```python
from build123d import *

# Parameters (mm, degrees)
EXTRUDE_1_DEPTH     = 20
SKETCH_2_W          = 12.3
SKETCH_2_H          = 5
CUT_EXTRUDE_1_DEPTH = 12
FILLET_1_R          = 1
FILLET_2_R          = 1.5
CUT_EXTRUDE_5_DEPTH = 21
SKETCH_3_R          = 0.9
CUT_EXTRUDE_2_DEPTH = 8
SKETCH_4_R          = 2
CUT_EXTRUDE_3_DEPTH = 8
CUT_EXTRUDE_4_DEPTH = 8


with BuildPart() as part:
    # 草图1 → 凸台-拉伸1 (new body)
    with BuildSketch(Plane(origin=(0, 0, 0), x_dir=(1, 0, 0), z_dir=(0, 1, 0))):
        with BuildLine():
            Line((-6.15, 0), (-11.5, 0))
            Line((-11.5, 0), (-11.5, 2))
            Line((-11.5, 2), (-8, 2))
            Line((-8, 2), (-8, 6.5))
            Line((-8, 6.5), (8, 6.5))
            Line((8, 6.5), (8, 2))
            Line((8, 2), (11.5, 2))
            Line((11.5, 2), (11.5, 0))
            Line((11.5, 0), (6.15, 0))
            ThreePointArc((6.15, 0), (5.470134317, 2.810717088), (3.580851854, 5))
            Line((3.580851854, 5), (-3.580851854, 5))
            ThreePointArc((-3.580851854, 5), (-5.470134317, 2.810717088), (-6.15, 0))
        make_face()
    extrude(amount=EXTRUDE_1_DEPTH)

    # 草图2 → 切除-拉伸1 (cut)
    with BuildSketch(Plane(origin=(0, 20, 0), x_dir=(1, 0, 0), z_dir=(0, 1, 0))):
        with Locations((0, 2.5)):
            Rectangle(SKETCH_2_W, SKETCH_2_H)
    extrude(amount=-CUT_EXTRUDE_1_DEPTH, mode=Mode.SUBTRACT)

    # 圆角1
    fillet_1_edges = [part.edges().sort_by_distance(p)[0] for p in [
        (-6.15, 14, -5),
        (6.15, 14, -5),
    ]]
    fillet(fillet_1_edges, radius=FILLET_1_R)

    # 圆角2
    fillet_2_edges = [part.edges().sort_by_distance(p)[0] for p in [
        (-8, 10, -2),
        (8, 10, -2),
    ]]
    fillet(fillet_2_edges, radius=FILLET_2_R)

    # 草图6 → 切除-拉伸5 (cut, through all)
    with BuildSketch(Plane(origin=(0, 20, 0), x_dir=(1, 0, 0), z_dir=(0, 1, 0))):
        Polygon((-5.75, 6.5), (-8.528510242, 4.895826364), (-8.528510242, 6.5), align=None)
        Polygon((8.528510242, 6.5), (5.75, 6.5), (8.528510242, 4.895826364), align=None)
    extrude(amount=-CUT_EXTRUDE_5_DEPTH, mode=Mode.SUBTRACT)

    # 草图3 → 切除-拉伸2 (cut)
    with BuildSketch(Plane(origin=(0, 0, -6.5), x_dir=(-1, 0, 0), z_dir=(0, 0, -1))):
        with Locations((-8, 4.5)):
            Circle(SKETCH_3_R)
        with Locations((-8, 15.5)):
            Circle(SKETCH_3_R)
        with Locations((8, 15.5)):
            Circle(SKETCH_3_R)
        with Locations((8, 4.5)):
            Circle(SKETCH_3_R)
    extrude(amount=-CUT_EXTRUDE_2_DEPTH, mode=Mode.SUBTRACT)

    # 草图4 → 切除-拉伸3 (cut)
    with BuildSketch(Plane(origin=(0, 0, -2), x_dir=(-1, 0, 0), z_dir=(0, 0, -1))):
        with Locations((-8, 15.5)):
            Circle(SKETCH_4_R)
        with Locations((-8, 4.5)):
            Circle(SKETCH_4_R)
        with Locations((8, 15.5)):
            Circle(SKETCH_4_R)
        with Locations((8, 4.5)):
            Circle(SKETCH_4_R)
    extrude(amount=CUT_EXTRUDE_3_DEPTH, mode=Mode.SUBTRACT)

    # 草图5 → 切除-拉伸4 (cut)
    with BuildSketch(Plane.XY.offset(-5)):
        with BuildLine():
            Line((-2.5, 17.5), (2.5, 17.5))
            ThreePointArc((2.5, 17.5), (3.207106781, 17.207106781), (3.5, 16.5))
            Line((3.5, 16.5), (3.5, 12.5))
            ThreePointArc((3.5, 12.5), (3.207106781, 11.792893219), (2.5, 11.5))
            Line((2.5, 11.5), (-2.5, 11.5))
            ThreePointArc((-2.5, 11.5), (-3.207106781, 11.792893219), (-3.5, 12.5))
            Line((-3.5, 12.5), (-3.5, 16.5))
            ThreePointArc((-3.5, 16.5), (-3.207106781, 17.207106781), (-2.5, 17.5))
        make_face()
    extrude(amount=-CUT_EXTRUDE_4_DEPTH, mode=Mode.SUBTRACT)


solid = part.part
```
Model file for the job. Use its own axes, mm. A direction names the side the tool comes from. Round coordinates to 2 decimals unless told otherwise and drop trailing zeros. Loops run counter-clockwise (first coordinate to the right, second up) from the corner with the lowest first, then second, coordinate; pieces in that order, holes last. Notation, with made-up numbers: M 83.25,79.5 L 96.25,79.5 A25 cw 96.25,103.5 Z; hole C -38.75,22.5 d5. An arc over 180 degrees is marked long. Put each result on its own line as item: value. Start each with the question number.
Item 1: Mould opens along X. For faces 1 (the face through (5.49, 3.94, -2.77)), 2 (the face through (-9, 10, 0)), 3 (the face through (-8.45, 1.26, -2.43)) say: released by +X, released by -X, zero draft, split by the parting line, or undercut.
Item 2: Drop flat-ended pins along their axis: P1, Ø3, axis at x = 8, y = 4.5, coming from the -Z side; P2, Ø1.4, axis at y = 8.5, z = -4, coming from the -X side; P3, Ø0.9, axis at y = 11, z = -4.5, coming from the +X side. Give the stop position or say it passes through.
Item 3: 3-axis set-ups, long thin cutter, end or side, ignore diameter. For faces 4 (the face through (-3.215, 17.199, -5.74)), 5 (the face through (-8, 10, -4)), 6 (the face through (-5.849, 13.916, -4.715)), 7 (the face through (8.43, 1.26, -2.45)): which of +Z, -Z, +X, -X, +Y, -Y reach the whole face in a straight line?
Item 4: Drill centre lines: line 1 along Y through (x, z) = (-8, -0.4); line 2 along Y through (x, z) = (8, -3); line 3 along X through (y, z) = (14, -0.5). Where is each one in solid material? Low to high.
Item 5: Cut at C-C (y = 15.5). List the corners of the cut face in (x, z), then the cut area to 3 significant figures.
Item 6: Cut at D-D (x = -8.25). List the corners of the cut face in (y, z).
Item 7: Cut at B-B (z = -1). List the corners of the cut face in (x, y), then the cut area to 3 significant figures.
Item 8: Cut at A-A (x = -1.5). List the corners of the cut face in (y, z), then the cut area to 3 significant figures.
Answer block:
1. face 1: undercut
1. face 2: zero draft
1. face 3: released by -X
2. P1: z = -2
2. P2: x = -8.01
2. P3: x = 8
3. face 4: +Z, -Z
3. face 5: -Z, -X, +Y, -Y
3. face 6: +Z, +Y
3. face 7: -Z, +X, +Y, -Y
4. line 1: 0 to 3.6, 5.4 to 14.6, 16.4 to 20
4. line 2: 0 to 2.5, 6.5 to 13.5, 17.5 to 20
4. line 3: -11.5 to -6.15, 6.15 to 11.5
5. outline: M -11.5,-2 L -8.9,-2 L -8.9,0 L -11.5,0 Z; M -7.1,-2 L -6.15,-2 L -6.15,0 L -7.1,0 Z; M -6,-6.36 L -5.75,-6.5 L -3.5,-6.5 L -3.5,-5 L -5.15,-5 A1 cw -6,-4.53 Z; M 3.5,-6.5 L 5.75,-6.5 L 6,-6.36 L 6,-4.53 A1 cw 5.15,-5 L 3.5,-5 Z; M 6.15,-2 L 7.1,-2 L 7.1,0 L 6.15,0 Z; M 8.9,-2 L 11.5,-2 L 11.5,0 L 8.9,0 Z
5. area: 21.9 mm2
6. outline: M 0,-2.67 L 2.52,-2.67 L 2.52,-2 L 3.64,-2 L 3.64,0 L 0,0 Z; M 5.36,-2 L 6.48,-2 L 6.48,-2.67 L 13.52,-2.67 L 13.52,-2 L 14.64,-2 L 14.64,0 L 5.36,0 Z; M 16.36,-2 L 17.48,-2 L 17.48,-2.67 L 20,-2.67 L 20,0 L 16.36,0 Z
7. outline: M -11.5,0 L -6.07,0 L -6.07,8 L -6.15,8 L -6.15,20 L -11.5,20 Z; M 6.07,0 L 11.5,0 L 11.5,20 L 6.15,20 L 6.15,8 L 6.07,8 Z; hole C -8,4.5 d1.8; hole C -8,15.5 d1.8; hole C 8,4.5 d1.8; hole C 8,15.5 d1.8
7. area: 205 mm2
8. outline: M 0,-6.5 L 11.5,-6.5 L 11.5,-5 L 0,-5 Z; M 17.5,-6.5 L 20,-6.5 L 20,-5 L 17.5,-5 Z
8. area: 21.0 mm2
